Part model, mm, in its own coordinate system. Face numbers are marked on the shaded views. A direction names the side the tool comes from. Give positions to 0.01 mm unless a question says otherwise; leave off trailing zeros. Write each loop counter-clockwise with the first axis right and the second up, starting at its lowest first coordinate (ties: lowest second). Pieces come first, ordered by that corner, then holes. Notation, with made-up numbers: M -34.5,65.25 L -17.5,65.25 A13 ccw -17.5,86.25 Z; hole C 61,45.5 d7. An arc over 180 degrees is marked long. Answer as CSV lines item,"result". Start each with the question number.
1) Tool access for the marked faces 1 and 2: list every direction of +Z, -Z, +X, -X, +Y, -Y with a clear straight run to the whole face (end or side of a thin tool).
2) Slice it at C-C, the plane y = -12. Give the cut face in (x, z), plus the area to 3 significant figures.
3) Slice it at A-A, the plane z = 8.5. Give the cut face in (x, y).
4) Pin check, flat tips, straight feed: pin 1 Ø9 at (y, z) = (-0.5, 10.5) entering from -X; pin 2 Ø9.5 at (y, z) = (7.5, 9.5) entering from -X; pin 3 Ø3 at (x, y) = (1.5, -8) entering from +Z. Stop position of each tip, or through.
5) Slice it at B-B, the plane x = -9.5. Give the cut face in (y, z).
6) Wall check: line 1 along X through (y, z) = (2, 10.75); line 2 along Z through (x, y) = (-18, -12.5); line 3 along Z through (x, y) = (21.5, 9.5). Give the ranges that are in metal, low to high. Write a range as from..to.
```python
from build123d import *

# Parameters (mm, degrees)
F0_W     = 60
F0_H     = 30
F1_DEPTH = 5
F2_W     = 5
F2_H     = 30
F3_DEPTH = 12
F4_SIZE  = 1
F5_SIZE  = 0.5


with BuildPart() as f1:
    # F0 (on Top) → F1 (new body)
    with BuildSketch(Plane.XY):
        Rectangle(F0_W, F0_H)
    extrude(amount=F1_DEPTH)

    # F2 (on face) → F3 (join)
    with BuildSketch(Plane.XY.offset(5)):
        with Locations((19.3, 0)):
            Rectangle(F2_W, F2_H)
        with Locations((27.5, 0)):
            Rectangle(F2_W, F2_H)
    extrude(amount=F3_DEPTH)

    # F4
    f4_edges = [f1.edges().sort_by_distance(p)[0] for p in [
        (21.8, 0, 17),
        (25, 0, 17),
    ]]
    chamfer(f4_edges, length=F4_SIZE)

    # F5
    f5_edges = [f1.edges().sort_by_distance(p)[0] for p in [
        (-6.6, -15, 5),
        (-30, 0, 5),
        (-6.6, 15, 5),
        (-30, -15, 2.5),
        (0, -15, 0),
        (23.4, -15, 5),
        (30, 0, 0),
        (16.8, 0, 17),
        (30, 0, 17),
        (-30, 0, 0),
        (30, -15, 8.5),
        (30, 15, 8.5),
        (23.4, 15, 5),
        (21.8, 15, 10.5),
        (25, 15, 10.5),
        (25, -15, 10.5),
        (21.8, -15, 10.5),
    ]]
    chamfer(f5_edges, length=F5_SIZE)


solid = f1.part
```
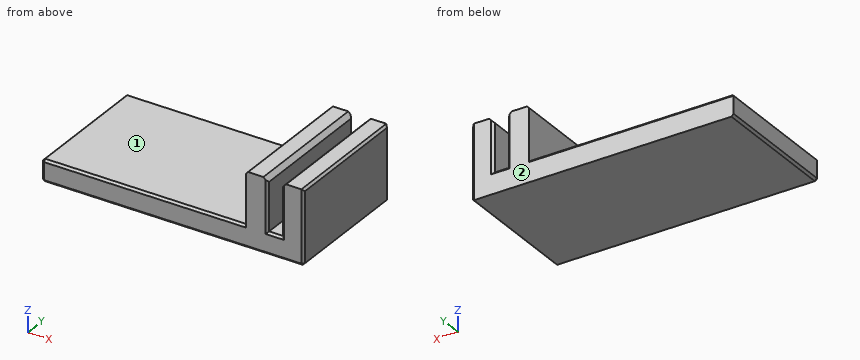
Found:
1,face 1,"+Z, -X, +Y, -Y"
1,face 2,"+Z, -Z, +X, -X, +Y"
2,outline,"M -30,0.5 L -29.5,0 L 29.5,0 L 30,0.5 L 30,16.5 L 29.5,17 L 26,17 L 25,16 L 25,5 L 21.8,5 L 21.8,16 L 20.8,17 L 17.3,17 L 16.8,16.5 L 16.8,5 L -29.5,5 L -30,4.5 Z"
2,area,"418 mm²"
3,outline,"M 16.8,-15 L 21.3,-15 L 21.8,-14.5 L 21.8,14.5 L 21.3,15 L 16.8,15 Z; M 25,-14.5 L 25.5,-15 L 29.5,-15 L 30,-14.5 L 30,14.5 L 29.5,15 L 25.5,15 L 25,14.5 Z"
4,pin 1,"x = 16.8"
4,pin 2,"x = -29.75"
4,pin 3,"z = 5"
5,outline,"M -15,0.5 L -14.5,0 L 15,0 L 15,4.5 L 14.5,5 L -14.5,5 L -15,4.5 Z"
6,line 1,"16.8..21.8, 25..30"
6,line 2,"0..5"
6,line 3,"0..16.3"
